Read the model definition and answer for the solid it produces. Units are mm, in the model's axes. Give positions to 0.01 mm unless a question says otherwise; leave off trailing zeros. Loops run counter-clockwise (first coordinate to the right, second up) from the corner with the lowest first, then second, coordinate; pieces in that order, holes last. Notation, with made-up numbers: (-32.75, 79.5) -> (-4.75, 79.5) arc R21 ccw to (-4.75, 116.5) -> close; hole circle Ø7 at (-11.5, 20). An arc over 180 degrees is marked (long way). Return JSON: item names as keys, results as strings. Group by question number.
from build123d import *

# Parameters (mm, degrees)
F1_DEPTH = 4


with BuildPart() as f1:
    # F0 (on Top) → F1 (new body)
    with BuildSketch(Plane.XY):
        with BuildLine():
            Line((-50, 50), (-50, 25))
            ThreePointArc((-50, 25), (-49.2383992871, 31.123724357), (-47, 36.874342087))
            Line((-47, 36.874342087), (-47, 47))
            Line((-47, 47), (-36.874342087, 47))
            ThreePointArc((-36.874342087, 47), (-31.123724357, 49.2383992871), (-25, 50))
            Line((-25, 50), (-50, 50))
        make_face()
        with BuildLine():
            ThreePointArc((-47, 36.874342087), (-49.2383992871, 31.123724357), (-50, 25))
            ThreePointArc((-50, 25), (-49.2383992871, 18.876275643), (-47, 13.125657913))
            Line((-47, 13.125657913), (-47, 25))
            Line((-47, 25), (-47, 36.874342087))
        make_face()
        with BuildLine():
            Line((-50, 0), (-25, 0))
            ThreePointArc((-25, 0), (-31.123724357, 0.7616007129), (-36.874342087, 3))
            Line((-36.874342087, 3), (-47, 3))
            Line((-47, 3), (-47, 13.125657913))
            ThreePointArc((-47, 13.125657913), (-49.2383992871, 18.876275643), (-50, 25))
            Line((-50, 25), (-50, 0))
        make_face()
        with BuildLine():
            ThreePointArc((-36.874342087, 3), (-31.123724357, 0.7616007129), (-25, 0))
            ThreePointArc((-25, 0), (-18.876275643, 0.7616007129), (-13.125657913, 3))
            Line((-13.125657913, 3), (-25, 3))
            Line((-25, 3), (-36.874342087, 3))
        make_face()
        with BuildLine():
            Line((-25, 0), (0, 0))
            Line((0, 0), (0, 25))
            ThreePointArc((0, 25), (-0.7616007129, 18.876275643), (-3, 13.125657913))
            Line((-3, 13.125657913), (-3, 3))
            Line((-3, 3), (-13.125657913, 3))
            ThreePointArc((-13.125657913, 3), (-18.876275643, 0.7616007129), (-25, 0))
        make_face()
        with BuildLine():
            ThreePointArc((-3, 13.125657913), (-0.7616007129, 18.876275643), (0, 25))
            ThreePointArc((0, 25), (-0.7616007129, 31.123724357), (-3, 36.874342087))
            Line((-3, 36.874342087), (-3, 25))
            Line((-3, 25), (-3, 13.125657913))
        make_face()
        with BuildLine():
            ThreePointArc((-3, 36.874342087), (-0.7616007129, 31.123724357), (0, 25))
            Line((0, 25), (0, 50))
            Line((0, 50), (-25, 50))
            ThreePointArc((-25, 50), (-18.876275643, 49.2383992871), (-13.125657913, 47))
            Line((-13.125657913, 47), (-3, 47))
            Line((-3, 47), (-3, 36.874342087))
        make_face()
        with BuildLine():
            ThreePointArc((-13.125657913, 47), (-18.876275643, 49.2383992871), (-25, 50))
            ThreePointArc((-25, 50), (-31.123724357, 49.2383992871), (-36.874342087, 47))
            Line((-36.874342087, 47), (-25, 47))
            Line((-25, 47), (-13.125657913, 47))
        make_face()
        with BuildLine():
            ThreePointArc((-36.874342087, 47), (-42.6776695297, 42.6776695297), (-47, 36.874342087))
            Line((-47, 36.874342087), (-47, 25))
            ThreePointArc((-47, 25), (-40.5563491861, 40.5563491861), (-25, 47))
            Line((-25, 47), (-36.874342087, 47))
        make_face()
        with BuildLine():
            ThreePointArc((-47, 13.125657913), (-42.6776695297, 7.3223304703), (-36.874342087, 3))
            Line((-36.874342087, 3), (-25, 3))
            ThreePointArc((-25, 3), (-40.5563491861, 9.4436508139), (-47, 25))
            Line((-47, 25), (-47, 13.125657913))
        make_face()
        with BuildLine():
            Line((-25, 3), (-13.125657913, 3))
            ThreePointArc((-13.125657913, 3), (-7.3223304703, 7.3223304703), (-3, 13.125657913))
            Line((-3, 13.125657913), (-3, 25))
            ThreePointArc((-3, 25), (-9.4436508139, 9.4436508139), (-25, 3))
        make_face()
        with BuildLine():
            Line((-3, 25), (-3, 36.874342087))
            ThreePointArc((-3, 36.874342087), (-7.3223304703, 42.6776695297), (-13.125657913, 47))
            Line((-13.125657913, 47), (-25, 47))
            ThreePointArc((-25, 47), (-9.4436508139, 40.5563491861), (-3, 25))
        make_face()
    extrude(amount=F1_DEPTH)


solid = f1.part
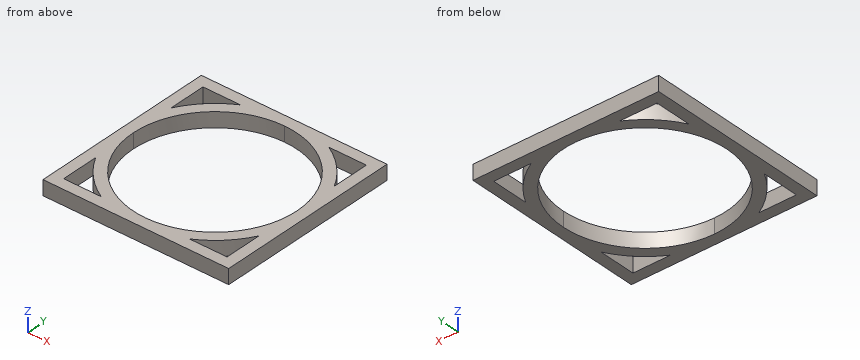
1. Section B-B on y = 38 is taken. Determine the outline of the cut face in (x, z), then the cut area to 3 significant figures.
2. Section A-A on x = -23.5 is taken. Determine the outline of the cut face in (y, z).
3. Straight lines are drawn through the part: line 1 (Y direction, x = -6, z = 3.45); line 2 (Y direction, x = -10.5, z = 1.35); line 3 (Y direction, x = -25.5, z = 2.45). For each, find the intervals that lie inside material, in ascending order. Write a range as from..to.
4. Section D-D on x = -4.5 is taken. Determine the outline of the cut face in (y, z).
5. Section C-C on z = 0.9 is taken. Determine the outline of the cut face in (x, y), then the cut area to 3 significant figures.
Completed:
{
 "1": {"outline": "(-50, 0) -> (-47, 0) -> (-47, 4) -> (-50, 4) -> close; (-46.35, 0) -> (-42.75, 0) -> (-42.75, 4) -> (-46.35, 4) -> close; (-7.25, 0) -> (-3.65, 0) -> (-3.65, 4) -> (-7.25, 4) -> close; (-3, 0) -> (0, 0) -> (0, 4) -> (-3, 4) -> close", "area": "52.8 mm²"},
 "2": {"outline": "(0, 0) -> (3.05, 0) -> (3.05, 4) -> (0, 4) -> close; (46.95, 0) -> (50, 0) -> (50, 4) -> (46.95, 4) -> close"},
 "3": {"line 1": "y = 0..3, 8.75..13.91, 36.09..41.25, 47..50", "line 2": "y = 0..3, 4.63..8.45, 41.55..45.37, 47..50", "line 3": "y = 0..3.01, 46.99..50"},
 "4": {"outline": "(0, 0) -> (3, 0) -> (3, 4) -> (0, 4) -> close; (10.69, 0) -> (17.02, 0) -> (17.02, 4) -> (10.69, 4) -> close; (32.98, 0) -> (39.31, 0) -> (39.31, 4) -> (32.98, 4) -> close; (47, 0) -> (50, 0) -> (50, 4) -> (47, 4) -> close"},
 "5": {"outline": "(-50, 0) -> (0, 0) -> (0, 50) -> (-50, 50) -> close; hole (-47, 3) -> (-36.87, 3) arc R25 cw to (-47, 13.13) -> close; hole circle Ø44 at (-25, 25); hole (-47, 36.87) arc R25 cw to (-36.87, 47) -> (-47, 47) -> close; hole (-13.13, 3) -> (-3, 3) -> (-3, 13.13) arc R25 cw to start; hole (-13.13, 47) arc R25 cw to (-3, 36.87) -> (-3, 47) -> close", "area": "815 mm²"}
}
